Geometry: final body of the model. Coordinates: model frame, mm. Face numbers are marked on the shaded views. A direction names the side the tool comes from. Coordinates: 2 decimals unless noted, no trailing zeros. Write each loop counter-clockwise with the first axis right and the second up, starting at its lowest first coordinate (ties: lowest second). Pieces come first, ordered by that corner, then holes. Notation, with made-up numbers: (16.25, 2) -> (34.25, 2) arc R22 cw to (34.25, 30) -> close; hole circle Ø5 at (-32.5, -25). An arc over 180 degrees is marked (long way). One line per item, written item: value.
```python
from build123d import *

# Parameters (mm, degrees)
F0_W      = 50.8
F0_H      = 50.8
F0_W_2    = 39.116
F0_H_2    = 39.116
F1_DEPTH  = 25.4
F2_W      = 50.8
F2_H      = 50.8
F3_DEPTH  = 25.4
F4_W      = 10.922
F4_H      = 8.255
F4_W_2    = 8.255
F4_H_2    = 10.922
F5_DEPTH  = 25.4
F6_R      = 7.62
F7_DEPTH  = 6.35
F8_SIZE2  = 15.24
F8_SIZE   = 5.08
F9_R      = 5.08
F10_SIZE2 = 1.27
F10_SIZE  = 10.16
F11_SIZE2 = 2.54
F11_SIZE  = 0.508
F12_R     = 1.27


with BuildPart() as f1:
    # F0 (on Top) → F1 (new body)
    with BuildSketch(Plane.XY):
        Rectangle(F0_W, F0_H)
        Rectangle(F0_W_2, F0_H_2, mode=Mode.SUBTRACT)
    extrude(amount=F1_DEPTH)

    # F2 (on face) → F3 (join)
    with BuildSketch(Plane(origin=(0, 0, 0), x_dir=(1, 0, 0), z_dir=(0, 0, -1))):
        Rectangle(F2_W, F2_H)
    extrude(amount=F3_DEPTH)

    # F4 (on face) → F5 (join)
    with BuildSketch(Plane.XY):
        with Locations((-14.097, 0)):
            Rectangle(F4_W, F4_H)
        with Locations((0, 14.097)):
            Rectangle(F4_W_2, F4_H_2)
        with Locations((14.097, 0)):
            Rectangle(F4_W, F4_H)
        with Locations((0, -14.097)):
            Rectangle(F4_W_2, F4_H_2)
    extrude(amount=F5_DEPTH)

    # F6 (on face) → F7 (cut)
    with BuildSketch(Plane.XY):
        Circle(F6_R)
    extrude(amount=-F7_DEPTH, mode=Mode.SUBTRACT)

    # F8
    f8_edges = [f1.edges().sort_by_distance(p)[0] for p in [
        (25.4, 0, -25.4),
        (0, -25.4, -25.4),
        (-25.4, 0, -25.4),
        (0, 25.4, -25.4),
    ]]
    f8_side = f1.faces().sort_by_distance((0, 0, -25.4))[0]
    chamfer(f8_edges, length=F8_SIZE, length2=F8_SIZE2, reference=f8_side)

    # F9
    f9_edges = [f1.edges().sort_by_distance(p)[0] for p in [
        (25.4, -25.4, 7.62),
        (25.4, 25.4, 7.62),
        (-25.4, 25.4, 7.62),
        (-25.4, -25.4, 7.62),
    ]]
    fillet(f9_edges, radius=F9_R)

    # F10
    f10_edges = [f1.edges().sort_by_distance(p)[0] for p in [
        (0, 25.4, 25.4),
    ]]
    f10_side = f1.faces().sort_by_distance((0, 25.4, 7.62))[0]
    chamfer(f10_edges, length=F10_SIZE, length2=F10_SIZE2, reference=f10_side)

    # F11
    f11_edges = [f1.edges().sort_by_distance(p)[0] for p in [
        (11.84275, -19.558, 25.4),
        (4.1275, -14.097, 25.4),
        (0, -8.636, 25.4),
        (-4.1275, -14.097, 25.4),
        (-11.84275, -19.558, 25.4),
        (-19.558, -11.84275, 25.4),
        (-14.097, -4.1275, 25.4),
        (-8.636, 0, 25.4),
        (-14.097, 4.1275, 25.4),
        (-19.558, 11.84275, 25.4),
        (-11.84275, 19.558, 25.4),
        (-4.1275, 14.097, 25.4),
        (0, 8.636, 25.4),
        (4.1275, 14.097, 25.4),
        (11.84275, 19.558, 25.4),
        (19.558, 11.84275, 25.4),
        (14.097, 4.1275, 25.4),
        (14.097, -4.1275, 25.4),
        (19.558, -11.84275, 25.4),
        (8.636, 0, 25.4),
    ]]
    chamfer(f11_edges, length=F11_SIZE, length2=F11_SIZE2)

    # F12
    f12_edges = [f1.edges().sort_by_distance(p)[0] for p in [
        (-19.558, 19.558, 11.43),
        (19.558, 19.558, 11.43),
        (19.558, -19.558, 11.43),
        (-19.558, -19.558, 11.43),
    ]]
    fillet(f12_edges, radius=F12_R)


solid = f1.part
```
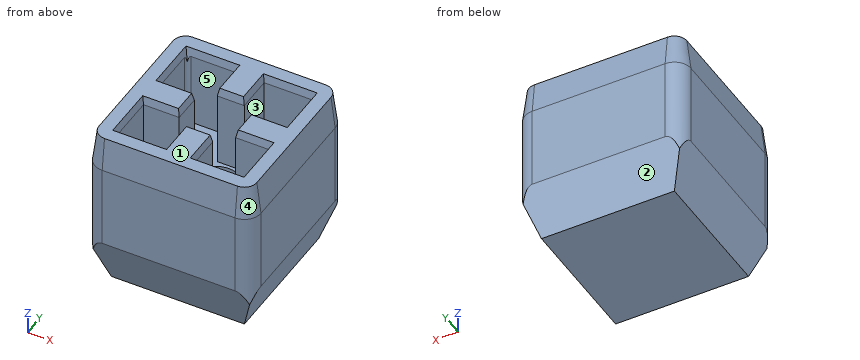
(1) Reachability of the marked faces 4 and 5 from +Z, -Z, +X, -X, +Y, -Y: full face, straight path, thin tool, end or side. Return the list, or none.
Responses:
face 4: +Z, +X, -Y
face 5: +Z
(2) Pull-direction query (Y, two-part tool) for the marked faces 1, 2 and 3; classes: released by +Y, released by -Y, zero draft, split by the parting line, or undercut.
Responses:
face 1: zero draft
face 2: released by +Y
face 3: undercut
(3) Section B-B (x = 0). Return the cut outline in (y, z), then the cut area to 3 significant figures.
Responses:
outline: (-25.4, -10.16) -> (-20.32, -25.4) -> (20.32, -25.4) -> (25.4, -10.16) -> (25.4, 15.24) -> (24.13, 25.4) -> (9.14, 25.4) -> (8.64, 22.86) -> (8.64, 0) -> (7.62, 0) -> (7.62, -6.35) -> (-7.62, -6.35) -> (-7.62, 0) -> (-8.64, 0) -> (-8.64, 22.86) -> (-9.14, 25.4) -> (-24.13, 25.4) -> (-25.4, 15.24) -> close
area: 1,950 mm2
(4) Line query: line 1 (X direction, y = 2, z = 8.5); line 2 (Y direction, x = 0, z = -1.25); line 3 (Z direction, x = -7, y = 10.5). Output: solid intervals per line, ascending. Write a range as [from, to].
Responses:
line 1: x = [-25.4, -8.64], [8.64, 25.4]
line 2: y = [-25.4, -7.62], [7.62, 25.4]
line 3: z = [-25.4, 0]
(5) Section D-D (z = -12). Return the cut outline in (x, y).
Responses:
outline: (-24.79, -22.74) arc R5.08 ccw to (-22.74, -24.79) -> (22.74, -24.79) arc R5.08 ccw to (24.79, -22.74) -> (24.79, 22.74) arc R5.08 ccw to (22.74, 24.79) -> (-22.74, 24.79) arc R5.08 ccw to (-24.79, 22.74) -> close
(6) First-contact query: pin 1 (2 mm diameter, centred on x = -4.5, z = -20, fed in from +Y); pin 2 (2 mm diameter, centred on x = -17.5, z = 20, fed in from -Y); pin 3 (12 mm diameter, centred on y = 12, z = 17.5, fed in from +X). Flat tips, straight axial feed; report the tip coordinate or a pass-through.
Responses:
pin 1: stops at y = 22.45
pin 2: stops at y = -24.93
pin 3: stops at x = 25.4
